from build123d import *

# Parameters (mm, degrees)
F0_W     = 10
F0_H     = 10
F0_R     = 1.75
F1_DEPTH = 6
F2_DEPTH = 4
F3_SIZE  = 1.9


with BuildPart() as f1:
    # F0 (on Top) → F1 (new body)
    with BuildSketch(Plane.XY):
        Rectangle(F0_W, F0_H)
        Polygon((-3.406367, 0), (-1.703183, 2.95), (1.703183, 2.95), (3.406367, 0), (1.703183, -2.95), (-1.703183, -2.95), align=None, mode=Mode.SUBTRACT)
        Polygon((1.703183, 2.95), (-1.703183, 2.95), (-3.406367, 0), (-1.703183, -2.95), (1.703183, -2.95), (3.406367, 0), align=None)
        Circle(F0_R, mode=Mode.SUBTRACT)
    extrude(amount=F1_DEPTH)

    # F0 (on Top) → F2 (cut)
    with BuildSketch(Plane.XY):
        Polygon((1.703183, 2.95), (-1.703183, 2.95), (-3.406367, 0), (-1.703183, -2.95), (1.703183, -2.95), (3.406367, 0), align=None)
        Circle(F0_R, mode=Mode.SUBTRACT)
    extrude(amount=F2_DEPTH, mode=Mode.SUBTRACT)

    # F3
    f3_edges = [f1.edges().sort_by_distance(p)[0] for p in [
        (0, 5, 0),
        (0, -5, 0),
        (0, 5, 6),
        (0, -5, 6),
    ]]
    chamfer(f3_edges, length=F3_SIZE)


solid = f1.part
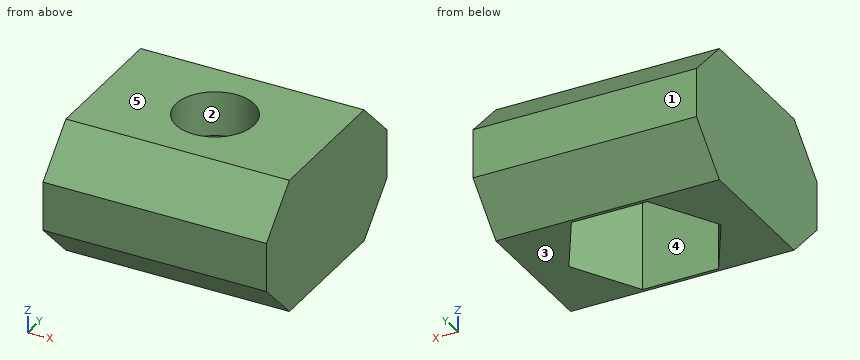
Here's how the part is built. I have some questions about the finished solid (model axes, mm). Face numbers are marked on the shaded views. A direction names the side the tool comes from. Coordinates: 2 decimals unless noted, no trailing zeros. Write each loop counter-clockwise with the first axis right and the second up, starting at its lowest first coordinate (ties: lowest second). Pieces come first, ordered by that corner, then holes.
1) I'm going to push flat-ended pins straight in: pin 1 (2 mm diameter, centred on x = 1.5, z = 5.5, fed in from -Y); pin 2 (1 mm diameter, centred on x = 3, z = 1, fed in from +Y). Where does each tip first touch, or does it pass through?
Filled in:
pin 1: stops at y = -4.6
pin 2: stops at y = 4.6
2) If I drill on line 1 (Y direction, x = -1.25, z = 3.25); line 2 (X direction, y = 1.25, z = 3); line 3 (Y direction, x = -0.75, z = 5.5), over which ranges is the centre line in solid material (lowest first)?
Filled in:
line 1: y = -5 to -2.95, 2.95 to 5
line 2: x = -5 to -2.68, 2.68 to 5
line 3: y = -3.6 to -1.58, 1.58 to 3.6
3) Thinking about a two-plate mould opening in Y: for the marked faces 1, 2 and 3, which applies, +Y half, -Y half, draft (parallel to the pull), parting line (faces both ways), or undercut?
Filled in:
face 1: +Y half
face 2: undercut
face 3: draft
4) If we section it at C-C (y = 1): List the corners of the cut face in (x, z) for me.
Filled in:
outline: (-5, 0) - (-2.83, 0) - (-2.83, 4) - (-1.44, 4) - (-1.44, 6) - (-5, 6) - close; (1.44, 4) - (2.83, 4) - (2.83, 0) - (5, 0) - (5, 6) - (1.44, 6) - close
5) If we section it at B-B (x = 0): List the corners of the cut face in (y, z) for me.
Filled in:
outline: (-5, 1.9) - (-3.1, 0) - (-2.95, 0) - (-2.95, 4) - (-1.75, 4) - (-1.75, 6) - (-3.1, 6) - (-5, 4.1) - close; (1.75, 4) - (2.95, 4) - (2.95, 0) - (3.1, 0) - (5, 1.9) - (5, 4.1) - (3.1, 6) - (1.75, 6) - close
6) If we section it at D-D (x = 3.75): List the corners of the cut face in (y, z) for me.
Filled in:
outline: (-5, 1.9) - (-3.1, 0) - (3.1, 0) - (5, 1.9) - (5, 4.1) - (3.1, 6) - (-3.1, 6) - (-5, 4.1) - close
7) If we section it at A-A (z = 3): List the corners of the cut face in (x, y) for me.
Filled in:
outline: (-5, -5) - (5, -5) - (5, 5) - (-5, 5) - close; hole (-3.41, 0) - (-1.7, -2.95) - (1.7, -2.95) - (3.41, 0) - (1.7, 2.95) - (-1.7, 2.95) - close
8) Which directions (+Z, -Z, +X, -X, +Y, -Y) give clear straight access to the entire face, cutting with the end or side of a thin tool? Please do the marked faces 4 and 5.
Filled in:
face 4: -Z
face 5: +Z, +X, -X, +Y, -Y
